Read the model definition and answer for the solid it produces. Units are mm, in the model's axes. A direction names the side the tool comes from. Coordinates: 2 decimals unless noted, no trailing zeros. Order: outer loops, then holes, each group sorted by start corner. A loop starts at its lowest first (then second) coordinate and runs counter-clockwise, first axis right, second up. Notation, with made-up numbers: M 34,85.25 L 63,85.25 A8 ccw 63,97.25 Z; hole C 65.5,38 d1. An arc over 180 degrees is marked long. Write each question's results on one line, items separated by ' | '.
```python
from build123d import *

# Parameters (mm, degrees)
BOSS_EXTRUDE1_DEPTH      = 10
BOSS_EXTRUDE1_DEPTH_BACK = 10
SKETCH1_W                = 40
SKETCH1_H                = 40.5
SKETCH2_W                = 20
SKETCH2_H                = 3
BOSS_EXTRUDE2_DEPTH      = 8
SKETCH3_W                = 20
SKETCH3_H                = 3
BOSS_EXTRUDE3_DEPTH      = 8
SKETCH4_R                = 2.5
BOSS_EXTRUDE4_DEPTH      = 4.5
SHELL1_T                 = -1
SKETCH5_R                = 2.1
CUT_EXTRUDE1_DEPTH       = 10
SKETCH6_R                = 2.1
CUT_EXTRUDE2_DEPTH       = 10


with BuildPart() as part:
    # Sketch1 → Boss-Extrude1 (new, two sides: drawn at the far end of the back side and taken through both)
    with BuildSketch(Plane.XY.offset(-BOSS_EXTRUDE1_DEPTH_BACK)):
        with Locations((20, 20.25)):
            Rectangle(SKETCH1_W, SKETCH1_H)
    extrude(amount=BOSS_EXTRUDE1_DEPTH + BOSS_EXTRUDE1_DEPTH_BACK)

    # Sketch2 → Boss-Extrude2 (add)
    with BuildSketch(Plane(origin=(40, 0, 0), x_dir=(0, 0, -1), z_dir=(1, 0, 0))):
        with Locations((0, 29)):
            Rectangle(SKETCH2_W, SKETCH2_H)
    extrude(amount=BOSS_EXTRUDE2_DEPTH)

    # Sketch3 → Boss-Extrude3 (add)
    with BuildSketch(Plane.ZY):
        with Locations((0, 29)):
            Rectangle(SKETCH3_W, SKETCH3_H)
    extrude(amount=BOSS_EXTRUDE3_DEPTH)

    # Sketch4 → Boss-Extrude4 (add)
    with BuildSketch(Plane(origin=(0, 40.5, 0), x_dir=(1, 0, 0), z_dir=(0, 1, 0))):
        with Locations((8.5, 0)):
            Circle(SKETCH4_R)
    extrude(amount=BOSS_EXTRUDE4_DEPTH)

    # Shell1
    shell1_openings = [part.faces().sort_by_distance(p)[0] for p in [
        (8.5, 45, 0),
    ]]
    offset(amount=SHELL1_T, openings=shell1_openings, kind=Kind.INTERSECTION)

    # Sketch5 → Cut-Extrude1 (cut)
    with BuildSketch(Plane(origin=(0, 30.5, 0), x_dir=(1, 0, 0), z_dir=(0, 1, 0))):
        with Locations((-6, 5.9)):
            Circle(SKETCH5_R)
        with Locations((-6, -5.9)):
            Circle(SKETCH5_R)
    extrude(amount=-CUT_EXTRUDE1_DEPTH, mode=Mode.SUBTRACT)

    # Sketch6 → Cut-Extrude2 (cut)
    with BuildSketch(Plane(origin=(0, 30.5, 0), x_dir=(1, 0, 0), z_dir=(0, 1, 0))):
        with Locations((46, 5.9)):
            Circle(SKETCH6_R)
        with Locations((46, -5.9)):
            Circle(SKETCH6_R)
    extrude(amount=-CUT_EXTRUDE2_DEPTH, mode=Mode.SUBTRACT)


solid = part.part
```
(1) The part is cut by section A-A, the plane z = -5.9. Write down the section's boundary in (x, y).
Conclusion:
outline: M -3.9,27.5 L 0,27.5 L 0,0 L 40,0 L 40,27.5 L 43.9,27.5 L 43.9,28.5 L 39,28.5 L 39,1 L 1,1 L 1,28.5 L -3.9,28.5 Z; M -3.9,29.5 L 1,29.5 L 1,39.5 L 39,39.5 L 39,29.5 L 43.9,29.5 L 43.9,30.5 L 40,30.5 L 40,40.5 L 0,40.5 L 0,30.5 L -3.9,30.5 Z
(2) The mould has two halves that part along X. Classify faces 1 (the flat face through (-8, 29, 8)), 2 (the cylindrical face through (-7.654, 29.021, -7.194)), 3 (the flat face through (42, 28.5, 0)), 4 (the flat face through (20, 21, -10)): pulls with the +X half, pulls with the -X half, needs draft (parallel to the pull), parting line crosses it, or undercut.
Conclusion:
face 1: pulls with the -X half | face 2: undercut | face 3: undercut | face 4: needs draft
(3) The part is cut by section D-D, the plane y = 4. Write down the section's boundary in (x, z), then the cut area to 3 significant figures.
Conclusion:
outline: M 0,-10 L 40,-10 L 40,10 L 0,10 Z; hole M 1,-9 L 39,-9 L 39,9 L 1,9 Z | area: 116 mm²
(4) The part is cut by section B-B, the plane x = 18.5. Write down the section's boundary in (y, z), then the cut area to 3 significant figures.
Conclusion:
outline: M 0,-10 L 40.5,-10 L 40.5,10 L 0,10 Z; hole M 1,-9 L 39.5,-9 L 39.5,9 L 1,9 Z | area: 117 mm²
(5) The part is cut by section C-C, the plane x = 46. Write down the section's boundary in (y, z), then the cut area to 3 significant figures.
Conclusion:
outline: M 27.5,-10 L 30.5,-10 L 30.5,-8 L 29.5,-8 L 29.5,-9 L 28.5,-9 L 28.5,-8 L 27.5,-8 Z; M 27.5,-3.8 L 28.5,-3.8 L 28.5,3.8 L 27.5,3.8 Z; M 27.5,8 L 28.5,8 L 28.5,9 L 29.5,9 L 29.5,8 L 30.5,8 L 30.5,10 L 27.5,10 Z; M 29.5,-3.8 L 30.5,-3.8 L 30.5,3.8 L 29.5,3.8 Z | area: 25.2 mm²
(6) Given pin 1 (5 mm diameter, centred on x = 46, z = -5.9, fed in from +Y); pin 2 (8 mm diameter, centred on y = 11.5, z = 0.5, fed in from -X); pin 3 (9 mm diameter, centred on x = -3, z = 1, fed in from +Y), each flat-ended and moving along its own axis, determine where each tip first touches the part or whether it passes through.
Conclusion:
pin 1: y = 30.5 | pin 2: x = 0 | pin 3: y = 40.5
(7) Straight lines are drawn through the part: line 1 (Z direction, x = -6, y = 28.3); line 2 (Y direction, x = 23, z = 8); line 3 (X direction, y = 26, z = 0). For each, find the intervals that lie inside material, in ascending order.
Conclusion:
line 1: -10 to -8, -3.8 to 3.8, 8 to 10 | line 2: 0 to 1, 39.5 to 40.5 | line 3: 0 to 1, 39 to 40
(8) For faces 5 (the flat face through (-3, 30.5, 0)), 6 (the flat face through (20, 21, -9)), 7 (the flat face through (0, 14, 0)), 8 (the flat face through (40, 35, 0)), determine the directions among +Z, -Z, +X, -X, +Y, -Y from which every point of the face is accessible in a straight line to the end or side of a thin tool.
Conclusion:
face 5: +Z, -Z, -X, +Y | face 6: none | face 7: +Z, -Z, -X, -Y | face 8: +Z, -Z, +X, +Y
